Can you work these out from the model? Positions are in its coordinate system, mm. Face numbers are marked on the shaded views. Give positions to 0.01 mm unless a question says otherwise; leave off trailing zeros. Order: outer loops, then holes, each group sorted by start corner. A loop starts at its lowest first (then second) coordinate and runs counter-clockwise, first axis right, second up. Notation, with made-up numbers: (3.25, 45.25) - (27.25, 45.25) arc R13 cw to (27.25, 61.25) - close; hole circle Ø2 at (52, 9.5). An arc over 180 degrees is marked (long way). Answer as a JSON object with one key per item and string values.
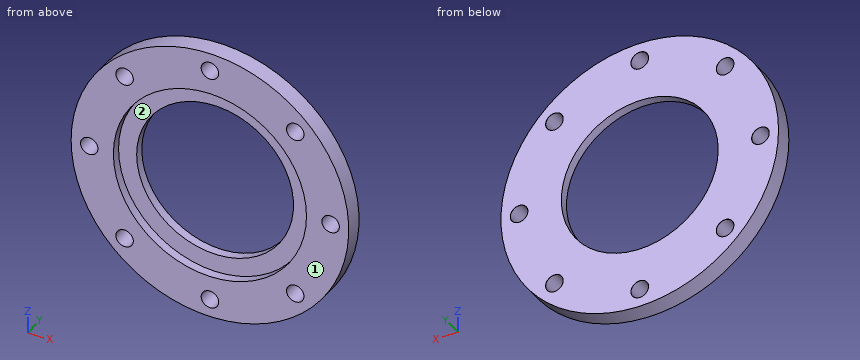
```python
from build123d import *

# Parameters (mm, degrees)
M5_CLEARANCE_HOLE1_D           = 5.8
M5_CLEARANCE_HOLE1_DEPTH       = 6
M5_CLEARANCE_HOLE1_CSINK_D     = 5.85
M5_CLEARANCE_HOLE1_CSINK_ANGLE = 90
CIRPATTERN1_COUNT              = 8


with BuildPart() as part:
    # Sketch1 → Revolve1 (revolve)
    with BuildSketch(Plane.XY):
        Polygon((-32, 0), (-46, 0), (-46, 6), (-26, 6), (-26, 3), (-32, 3), align=None)
    revolve(axis=Axis((0, 0, 0), (0, 1, 0)))

    # M5 Clearance Hole1
    with Locations(Plane(origin=(0, 6, 0), x_dir=(1, 0, 0), z_dir=(0, 1, 0))):
        with Locations((40, 0)):
            m5_clearance_hole1 = CounterSinkHole(M5_CLEARANCE_HOLE1_D / 2, M5_CLEARANCE_HOLE1_CSINK_D / 2, depth=M5_CLEARANCE_HOLE1_DEPTH, counter_sink_angle=M5_CLEARANCE_HOLE1_CSINK_ANGLE)

    # CirPattern1: M5 Clearance Hole1 ×8 about axis
    cirpattern1_axis = Axis((0, 0, 0), (0, 1, 0))
    for i in range(1, CIRPATTERN1_COUNT):
        add(m5_clearance_hole1.rotate(cirpattern1_axis, i * 360 / CIRPATTERN1_COUNT), mode=Mode.SUBTRACT)


solid = part.part
```
Q1. I'm going to push flat-ended pins straight in: pin 1 Ø1.5 at (y, z) = (2, -13) entering from -X; pin 2 Ø3 at (y, z) = (2.5, 22.5) entering from +X; pin 3 Ø10 at (x, z) = (-4.5, 26) entering from -Y. Where does each tip first touch, or does it pass through?
Recorded:
{"pin 1": "stops at x = -44.34", "pin 2": "stops at x = 40.93", "pin 3": "stops at y = 3"}
Q2. I need wall thicknesses on L1, parallel to X at y = 3.6, z = 27.5; L2, parallel to Z at x = -1, y = 5.05; L3, parallel to X at y = 5.45, z = -2. Which ranges of each line are inside material? Lowest first, please.
Recorded:
{"L1": "x = -36.87 to -31.08, -25.49 to 25.49, 31.08 to 36.87", "L2": "z = -45.99 to -42.72, -37.28 to -25.98, 25.98 to 37.28, 42.72 to 45.99", "L3": "x = -45.96 to -42.1, -37.9 to -25.92, 25.92 to 37.9, 42.1 to 45.96"}
Q3. We'd pull the mould along X, two halves only. Please class the marked faces 1 and 2: released by +X, released by -X, zero draft, split by the parting line, or undercut.
Recorded:
{"face 1": "zero draft", "face 2": "undercut"}
Q4. If we section it at B-B, the plane x = 0: Please give me the cut outline in (y, z) (3 decimals), then the cut area to 3 significant figures.
Recorded:
{"outline": "(0, -46) - (6, -46) - (6, -42.925) - (5.975, -42.9) - (0, -42.9) - close; (0, -37.1) - (5.975, -37.1) - (6, -37.075) - (6, -26) - (3, -26) - (3, -32) - (0, -32) - close; (0, 32) - (3, 32) - (3, 26) - (6, 26) - (6, 37.075) - (5.975, 37.1) - (0, 37.1) - close; (0, 42.9) - (5.975, 42.9) - (6, 42.925) - (6, 46) - (0, 46) - close", "area": "134 mm^2"}
Q5. If we section it at A-A, the plane z = 0: Please give me the cut outline in (x, y) (3 decimals).
Recorded:
{"outline": "(-46, 0) - (-42.9, 0) - (-42.9, 5.975) - (-42.925, 6) - (-46, 6) - close; (-37.1, 0) - (-32, 0) - (-32, 3) - (-26, 3) - (-26, 6) - (-37.075, 6) - (-37.1, 5.975) - close; (26, 3) - (32, 3) - (32, 0) - (37.1, 0) - (37.1, 5.975) - (37.075, 6) - (26, 6) - close; (42.9, 0) - (46, 0) - (46, 6) - (42.925, 6) - (42.9, 5.975) - close"}
Q6. If we section it at C-C, the plane z = -21.5: Please give me the cut outline in (x, y).
Recorded:
{"outline": "(-40.67, 0) - (-23.7, 0) - (-23.7, 3) - (-14.62, 3) - (-14.62, 6) - (-40.67, 6) - close; (14.62, 3) - (23.7, 3) - (23.7, 0) - (40.67, 0) - (40.67, 6) - (14.62, 6) - close"}
Q7. If we section it at D-D, the plane y = 1.05: Count the separate pieces of the cut face and the enclosed holes in it, then the cut area to 3 significant figures.
Recorded:
{"separate pieces": "1", "enclosed holes": "9", "area": "3,220 mm^2"}
